from build123d import *

# Parameters (mm, degrees)
PAD003_DEPTH         = 3
SKETCH012_R          = 0.5
POCKET003_DEPTH      = 16.301
POCKET003_DEPTH_BACK = 16.301
SKETCH013_W          = 30.27619
SKETCH013_H          = 27.7
POCKET004_DEPTH      = 1.5
SKETCH014_W          = 25.766444
SKETCH014_H          = 24.595242
POCKET005_DEPTH      = 3.001
FILLET_R             = 1.2
PAD005_DEPTH         = 5
FILLET002_R          = 2


with BuildPart() as part:
    # Sketch009 → Pad003 (new body)
    with BuildSketch(Plane.XY):
        Polygon((-11.8, 14.8), (-16.3, 14.8), (-16.3, -16.3), (16.3, -16.3), (16.3, 14.8), (11.8, 14.8), (11.8, 17.8), (-11.8, 17.8), align=None)
    extrude(amount=PAD003_DEPTH)

    # Sketch010 (on DatumPlane) → SubtractiveLoft section 0
    with BuildSketch(Plane.XZ.offset(16.5)):
        with BuildLine():
            ThreePointArc((-6, 2.25), (-6.75, 1.5), (-6, 0.75))
            Line((-6, 0.75), (6, 0.75))
            ThreePointArc((6, 0.75), (6.75, 1.5), (6, 2.25))
            Line((-6, 2.25), (6, 2.25))
        make_face()
    # Sketch011 (on DatumPlane) → SubtractiveLoft section 1
    with BuildSketch(Plane.XZ.offset(15.7)):
        with BuildLine():
            ThreePointArc((-3.75, 2), (-4.25, 1.5), (-3.75, 1))
            Line((-3.75, 1), (3.75, 1))
            ThreePointArc((3.75, 1), (4.25, 1.5), (3.75, 2))
            Line((-3.75, 2), (3.75, 2))
        make_face()
    loft(mode=Mode.SUBTRACT)

    # Sketch012 (on DatumPlane) → Pocket003 (cut, two sides)
    with BuildSketch(Plane.YZ) as pocket003_sk:
        with Locations((16.8, 1.5)):
            Circle(SKETCH012_R)
    extrude(amount=-POCKET003_DEPTH, mode=Mode.SUBTRACT)
    extrude(pocket003_sk.sketch, amount=POCKET003_DEPTH_BACK, mode=Mode.SUBTRACT)

    # Sketch013 (on DatumPlane) → Pocket004 (cut)
    with BuildSketch(Plane.XY.offset(3)):
        with Locations((0, -0.15)):
            Rectangle(SKETCH013_W, SKETCH013_H)
    extrude(amount=-POCKET004_DEPTH, mode=Mode.SUBTRACT)

    # Sketch014 (on DatumPlane) → Pocket005 (cut, through all)
    with BuildSketch(Plane.XY.offset(3)):
        with Locations((0, -0.75)):
            Rectangle(SKETCH014_W, SKETCH014_H)
    extrude(amount=-POCKET005_DEPTH, mode=Mode.SUBTRACT)

    # Fillet
    fillet_edges = [part.edges().sort_by_distance(p)[0] for p in [
        (0, 17.8, 3),
        (0, 17.8, 0),
    ]]
    fillet(fillet_edges, radius=FILLET_R)

    # Sketch018 (on DatumPlane) → Pad005 (join, symmetric)
    with BuildSketch(Plane.YZ):
        with BuildLine():
            Line((-14, 3), (-15, 3))
            add(Edge.make_bspline(
                [(-15, 3), (-14.589899, 4.698463), (-16.3, 5.5)],
                knots=[0, 0, 0, 1, 1, 1], degree=2))
            Line((-16.3, 5.5), (-16.3, 6.3))
            add(Edge.make_bspline(
                [(-14, 3), (-13.679767, 5.619108), (-16.3, 6.3)],
                knots=[0, 0, 0, 1, 1, 1], degree=2))
        make_face()
    extrude(amount=PAD005_DEPTH, both=True)

    # Fillet002
    fillet002_edges = [part.edges().sort_by_distance(p)[0] for p in [
        (16.3, -16.3, 1.5),
        (16.3, 14.8, 1.5),
        (-16.3, 14.8, 1.5),
        (-16.3, -16.3, 1.5),
    ]]
    fillet(fillet002_edges, radius=FILLET002_R)


with BuildPart() as part_1:
    # cover placement: moved
    add(part.part.moved(Location((0, 0, 55))))


solid = part_1.part
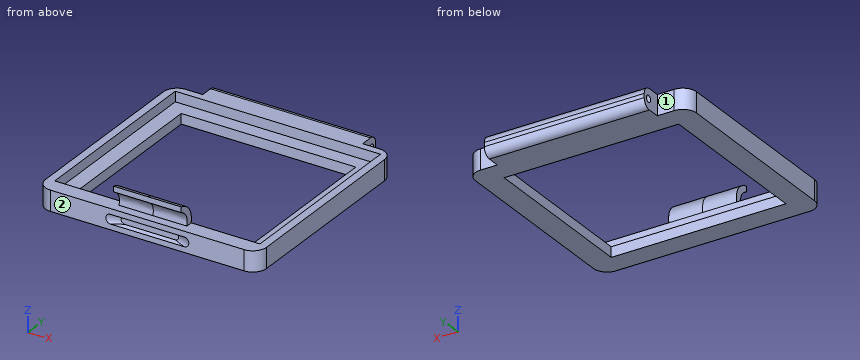
The listing builds one solid part. Answer for the finished solid, in the listing's coordinates (mm). Face numbers are marked on the shaded views. A direction names the side the tool comes from. Give positions to 0.01 mm unless a question says otherwise; leave off trailing zeros. Write each loop counter-clockwise with the first axis right and the second up, starting at its lowest first coordinate (ties: lowest second). Pieces come first, ordered by that corner, then holes. Notation, with made-up numbers: (-38, 40) - (-34, 40) arc R19 cw to (-34, 60) - close; hole circle Ø6 at (9.5, -5.5). An arc over 180 degrees is marked (long way). Use a Markdown table: item, result.
1. Find the intervals of material crossed by probe 1 along X at (y, z) = (-1.5, 55.5); probe 2 along Y at (x, z) = (-3, 56.75); probe 3 along X at (y, z) = (7.5, 57), in increasing order. Write a range as from..to.
Values follow:
| item | result |
|---|---|
| probe 1 | x = -16.3..-12.88, 12.88..16.3 |
| probe 2 | y = -15.7..-14, 13.7..16.37, 17.23..17.8 |
| probe 3 | x = -16.3..-15.14, 15.14..16.3 |
2. A tool of negligible diameter and unlimited length cuts with its end or side. For the marked faces 1 and 2, from which of +Z, -Z, +X, -X, +Y, -Y can it reach the whole face along a straight path? Write none if from no direction.
Values follow:
| item | result |
|---|---|
| face 1 | +Z, -Z, -X, +Y |
| face 2 | +Z, -Z, +X, -X, -Y |
3. Each of these flat-tipped pins is pushed along its axis until it touches: P1, Ø0.9, axis at y = 15.5, z = 57, coming from the +X side; P2, Ø0.8, axis at x = 12.5, z = 57, coming from the +Y side; P3, Ø2.5, axis at y = -15, z = 59, coming from the +X side; P4, Ø0.9, axis at y = 17, z = 57, coming from the -X side. Where does it stop, or does it pass through?
Values follow:
| item | result |
|---|---|
| P1 | stops at x = 11.8 |
| P2 | stops at y = 14.8 |
| P3 | stops at x = 16.3 |
| P4 | stops at x = -11.8 |
4. Section A-A on y = -9.5 is taken. Write down the section's boundary in (x, z).
Values follow:
| item | result |
|---|---|
| outline | (-16.3, 55) - (-12.88, 55) - (-12.88, 56.5) - (-15.14, 56.5) - (-15.14, 58) - (-16.3, 58) - close; (12.88, 55) - (16.3, 55) - (16.3, 58) - (15.14, 58) - (15.14, 56.5) - (12.88, 56.5) - close |
5. Section B-B on x = -0.5 is taken. Count the separate pieces of the cut face and the enclosed holes in it, plus the area to 3 significant figures.
Values follow:
| item | result |
|---|---|
| separate pieces | 2 |
| enclosed holes | 1 |
| area | 25.2 mm² |
